```python
from build123d import *

# Parameters (mm, degrees)
SKETCH1_W           = 107
SKETCH1_H           = 145
BOSS_EXTRUDE1_DEPTH = 3
SKETCH3_W           = 35
SKETCH3_H           = 3
BOSS_EXTRUDE4_DEPTH = 3
SKETCH4_W           = 35
SKETCH4_H           = 3
BOSS_EXTRUDE5_DEPTH = 3
SKETCH5_W           = 35
SKETCH5_H           = 3
BOSS_EXTRUDE6_DEPTH = 3
SKETCH6_W           = 35
SKETCH6_H           = 3
BOSS_EXTRUDE7_DEPTH = 3


with BuildPart() as part:
    # Sketch1 → Boss-Extrude1 (new body)
    with BuildSketch(Plane(origin=(0, 0, 0), x_dir=(1, 0, 0), z_dir=(0, 1, 0))):
        Rectangle(SKETCH1_W, SKETCH1_H)
    extrude(amount=BOSS_EXTRUDE1_DEPTH)

    # Sketch3 → Boss-Extrude4 (add)
    with BuildSketch(Plane(origin=(53.5, 0, 0), x_dir=(0, 0, -1), z_dir=(1, 0, 0))):
        with Locations((36.453510912, 1.5)):
            Rectangle(SKETCH3_W, SKETCH3_H)
        with Locations((-36.453510912, 1.5)):
            Rectangle(SKETCH3_W, SKETCH3_H)
    extrude(amount=BOSS_EXTRUDE4_DEPTH)

    # Sketch4 → Boss-Extrude5 (add)
    with BuildSketch(Plane.ZY.offset(53.5)):
        with Locations((-36.45, 1.5)):
            Rectangle(SKETCH4_W, SKETCH4_H)
        with Locations((36.45, 1.5)):
            Rectangle(SKETCH4_W, SKETCH4_H)
    extrude(amount=BOSS_EXTRUDE5_DEPTH)

    # Sketch5 → Boss-Extrude6 (add)
    with BuildSketch(Plane.XY.offset(72.5)):
        with Locations((0, 1.5)):
            Rectangle(SKETCH5_W, SKETCH5_H)
    extrude(amount=BOSS_EXTRUDE6_DEPTH)

    # Sketch6 → Boss-Extrude7 (add)
    with BuildSketch(Plane(origin=(0, 0, -72.5), x_dir=(-1, 0, 0), z_dir=(0, 0, -1))):
        with Locations((0, 1.5)):
            Rectangle(SKETCH6_W, SKETCH6_H)
    extrude(amount=BOSS_EXTRUDE7_DEPTH)


solid = part.part
```
Check sheet for the modelled part. Datum: model origin and axes. Units: mm. A direction names the side the tool comes from. Give positions to 0.01 mm unless a question says otherwise; leave off trailing zeros. Write each loop counter-clockwise with the first axis right and the second up, starting at its lowest first coordinate (ties: lowest second). Pieces come first, ordered by that corner, then holes.
Item 1: Cross-section at A-A (y = 1.95). Enter the section's corners in (x, z), and give its area (3 significant figures).
Item 2: Access from +Z, -Z, +X, -X, +Y, -Y to the whole of each face (thin tool, end or side, straight path). Record for faces 1 (the face through (55, 1, 53.954)), 2 (the face through (-53.5, 1, 63)), 3 (the face through (-53.5, 1, 0)), 4 (the face through (55, 1, -18.954)).
Item 3: Scan lines: L1, parallel to Z at x = 24, y = 2.55; L2, parallel to X at y = 2.4, z = 11.5. Record each from-to range of solid material in increasing order.
Item 4: Gauge pin test, flat ends, axial feed: pin 1 (0.9 mm diameter, centred on x = 55, y = 2, fed in from +Z); pin 2 (0.9 mm diameter, centred on y = 1.5, z = 63, fed in from +X); pin 3 (0.9 mm diameter, centred on x = -41.5, y = 1.5, fed in from -Z). Record the tip position at first contact, or that the pin passes through.
Item 5: Cross-section at B-B (z = -57). Enter the section's corners in (x, y).
Item 6: Draft check along Z on faces 5 (the face through (-55, 1, 18.95)), 6 (the face through (17.5, 1, -74)), 7 (the face through (0, 2, 75.5)). Enter one of: released by +Z, released by -Z, zero draft, split by the parting line, or undercut.
Item 7: Cross-section at C-C (x = 36.5). Enter the section's corners in (y, z).
Report:
1. outline: (-56.5, -53.95) - (-53.5, -53.95) - (-53.5, -72.5) - (-17.5, -72.5) - (-17.5, -75.5) - (17.5, -75.5) - (17.5, -72.5) - (53.5, -72.5) - (53.5, -53.95) - (56.5, -53.95) - (56.5, -18.95) - (53.5, -18.95) - (53.5, 18.95) - (56.5, 18.95) - (56.5, 53.95) - (53.5, 53.95) - (53.5, 72.5) - (17.5, 72.5) - (17.5, 75.5) - (-17.5, 75.5) - (-17.5, 72.5) - (-53.5, 72.5) - (-53.5, 53.95) - (-56.5, 53.95) - (-56.5, 18.95) - (-53.5, 18.95) - (-53.5, -18.95) - (-56.5, -18.95) - close
1. area: 16,100 mm2
2. face 1: +Z, +X, +Y, -Y
2. face 2: +Z, -X, +Y, -Y
2. face 3: -X, +Y, -Y
2. face 4: +X, +Y, -Y
3. L1: z = -72.5 to 72.5
3. L2: x = -53.5 to 53.5
4. pin 1: stops at z = 53.95
4. pin 2: stops at x = 53.5
4. pin 3: stops at z = -72.5
5. outline: (-53.5, 0) - (53.5, 0) - (53.5, 3) - (-53.5, 3) - close
6. face 5: undercut
6. face 6: zero draft
6. face 7: released by +Z
7. outline: (0, -72.5) - (3, -72.5) - (3, 72.5) - (0, 72.5) - close
